Design review of the part built by this model. Coordinates are the model's own, in mm. A direction names the side the tool comes from. Give positions to 0.01 mm unless a question says otherwise; leave off trailing zeros. Write each loop counter-clockwise with the first axis right and the second up, starting at its lowest first coordinate (ties: lowest second). Pieces come first, ordered by that corner, then holes. Notation, with made-up numbers: M 6,56 L 35,56 A19 cw 35,76 Z; hole C 55.25,-21 d7. An arc over 180 degrees is marked long. Answer in a Markdown table with one row per item.
```python
from build123d import *

# Parameters (mm, degrees)
F1_DEPTH = 3
F3_DEPTH = 2


with BuildPart() as f1:
    # F0 (on Top) → F1 (new body)
    with BuildSketch(Plane.XY):
        Polygon((-23.565747, 8.733586), (-26.811946, 7.810456), (-26.811946, -4.42697), (-24.105687, -5.435429), (-24.105687, 3.273411), (-21.755431, -6.025282), (-18.503955, -6.848847), (-18.503955, 9.736739), (-21.37113, 9.227031), (-21.37113, 0.183831), align=None)
        Polygon((-10.527196, 10.851217), (-17.061597, 9.973913), (-17.063336, -7.120089), (-10.348095, -8.144408), (-10.390801, -4.450301), (-14.086946, -4.170476), (-14.086946, -0.409178), (-10.908057, -0.372427), (-10.950724, 3.318271), (-14.086946, 3.318271), (-14.127168, 6.797468), (-10.484197, 7.131785), align=None)
        Polygon((-6.843771, 10.887864), (-10.013774, 10.851217), (-7.693077, -8.587812), (-4.531018, -8.831803), (-3.521484, 4.251498), (-2.791821, -8.831803), (0.67818, -8.791688), (2.618703, 8.953662), (2.700111, 7.121005), (4.679172, 7.143884), (4.679172, -8.443333), (7.66364, -8.408831), (7.66364, 7.143884), (9.612382, 7.166413), (9.569359, 10.887864), (0, 11.354624), (-1.080738, -2.574903), (-2.025757, 11.187691), (-4.974215, 11.153605), (-5.970521, -2.398258), align=None)
        Polygon((22.529045, 8.955718), (19.260596, 9.551114), (19.448553, -6.707126), (22.146616, -6.036957), (22.044722, 2.776925), (24.294013, -5.235689), (27.544877, -4.323111), (27.544877, 7.68314), (24.666015, 8.379457), (24.758457, 0.383226), align=None)
        with BuildLine():
            ThreePointArc((13.56484, 10.614374), (12.58338, 10.612468), (11.67815, 10.233224))
            ThreePointArc((11.67815, 10.233224), (10.567721, 8.708449), (10.191667, 6.860051))
            Line((10.191667, 6.860051), (10.194493, -3.856149))
            ThreePointArc((10.194493, -3.856149), (10.374655, -5.290787), (10.903246, -6.636608))
            ThreePointArc((10.903246, -6.636608), (11.635651, -7.532128), (12.656043, -8.077263))
            ThreePointArc((12.656043, -8.077263), (13.79671, -8.051781), (14.901063, -7.765121))
            ThreePointArc((14.901063, -7.765121), (16.071482, -7.074666), (17.002018, -6.084357))
            ThreePointArc((17.002018, -6.084357), (17.757929, -4.668834), (18.001225, -3.082671))
            Line((18.001225, -3.082671), (17.833713, 6.802879))
            ThreePointArc((17.833713, 6.802879), (17.166492, 8.640981), (15.767285, 10.007006))
            ThreePointArc((15.767285, 10.007006), (14.704057, 10.448465), (13.56484, 10.614374))
        make_face()
        with BuildLine():
            Line((13.219225, -3.660286), (13.219225, 6.444435))
            ThreePointArc((13.219225, 6.444435), (13.353404, 6.964312), (13.722419, 7.354317))
            ThreePointArc((13.722419, 7.354317), (14.10761, 7.367864), (14.448463, 7.187932))
            ThreePointArc((14.448463, 7.187932), (14.708863, 6.844124), (14.870914, 6.444435))
            Line((14.870914, 6.444435), (14.98508, -3.430936))
            ThreePointArc((14.98508, -3.430936), (14.798828, -4.132397), (14.277328, -4.637151))
            ThreePointArc((14.277328, -4.637151), (13.87296, -4.652777), (13.509215, -4.475443))
            ThreePointArc((13.509215, -4.475443), (13.293882, -4.092887), (13.219225, -3.660286))
        make_face(mode=Mode.SUBTRACT)
    extrude(amount=F1_DEPTH)

    # F2 (on face) → F3 (join)
    with BuildSketch(Plane(origin=(0, 0, 0), x_dir=(1, 0, 0), z_dir=(0, 0, -1))):
        with BuildLine():
            Line((29.726516, -9.49899), (29.907823, 6.184002))
            ThreePointArc((29.907823, 6.184002), (0.143357, 11.231437), (-29.651286, 6.365308))
            Line((-29.651286, 6.365308), (-29.46998, -9.227031))
            ThreePointArc((-29.46998, -9.227031), (0.106665, -14.06537), (29.726516, -9.49899))
        make_face()
    extrude(amount=F3_DEPTH)


solid = f1.part
```
1) The part is to be moulded in two halves that separate along Y. For faces 1 (the face through (-12.331, 6.962, 1.479)), 2 (the face through (-6.13, -8.71, 1.48)), 3 (the face through (13, 1, 3)), say which applies: released by +Y, released by -Y, zero draft, split by the parting line, or undercut.
Geometry says:
| item | result |
|---|---|
| face 1 | undercut |
| face 2 | released by -Y |
| face 3 | zero draft |
2) For faces 4 (the face through (20.92, 9.25, 1.48)), 5 (the face through (16.057, -7.087, 1.479)), 6 (the face through (25.897, -4.786, 1.479)), 7 (the face through (14, 1, 0)), 8 (the face through (27.545, 2, 1)), list the 3-axis set-ups (+Z, -Z, +X, -X, +Y, -Y) from which the entire face can be reached by the end or side of a thin tool; tool diameter is ignored.
Geometry says:
| item | result |
|---|---|
| face 4 | +Z, +X, +Y |
| face 5 | +Z, -Y |
| face 6 | +Z, +X, -Y |
| face 7 | +Z |
| face 8 | +Z, +X, +Y, -Y |
3) Add section A-A (z = 0.7). Count the separate pieces of the cut face and the enclosed holes in it, and give its area (3 significant figures).
Geometry says:
| item | result |
|---|---|
| separate pieces | 5 |
| enclosed holes | 1 |
| area | 648 mm^2 |
4) Add section C-C (x = 6). Write out the cut boundary in (y, z), and give its area (3 significant figures).
Geometry says:
| item | result |
|---|---|
| outline | M -11.03,-2 L 13.91,-2 L 13.91,0 L 11.06,0 L 11.06,3 L -8.43,3 L -8.43,0 L -11.03,0 Z |
| area | 108 mm^2 |
5) To check wall thickness, follow probe 1 along Y at (x, z) = (-12.5, 1.75); probe 2 along Z at (x, y) = (-14, -4); probe 3 along X at (y, z) = (7.75, -1.4). State the ranges of each line that lie inside material, in increasing order. Write a range as [from, to].
Geometry says:
| item | result |
|---|---|
| probe 1 | [-7.82, -4.29], [-0.39, 3.32], [6.95, 10.59] |
| probe 2 | [-2, 0] |
| probe 3 | [-29.49, 29.75] |
6) Add section B-B (x = -16.5). Write out the cut boundary in (y, z), and give its area (3 significant figures).
Geometry says:
| item | result |
|---|---|
| outline | M -9.76,-2 L 12.53,-2 L 12.53,0 L 10.05,0 L 10.05,3 L -7.21,3 L -7.21,0 L -9.76,0 Z |
| area | 96.4 mm^2 |
7) Insertion check: P1, Ø1.4, axis at x = 14, y = 2, coming from the +Z side; P2, Ø1.5, axis at y = -3.5, z = 1.5, coming from the +X side; P3, Ø1.5, axis at y = 3, z = 1, coming from the -X side. Each pin has a flat end and moves straight along its axis. Give the tip position at first contact, or say it passes through.
Geometry says:
| item | result |
|---|---|
| P1 | z = 0 |
| P2 | x = 27.54 |
| P3 | x = -26.81 |
